Build history of the part. All positions in model axes, mm. Face numbers are marked on the shaded views. A direction names the side the tool comes from. Round coordinates to 2 decimals unless told otherwise and drop trailing zeros. Write each loop counter-clockwise with the first axis right and the second up, starting at its lowest first coordinate (ties: lowest second). Pieces come first, ordered by that corner, then holes. Notation, with made-up numbers: M 36.5,3 L 46.5,3 A31 cw 46.5,36 Z; hole C -24.75,-37.5 d2. An arc over 180 degrees is marked long. One line per item, written item: value. Start each with the question number.
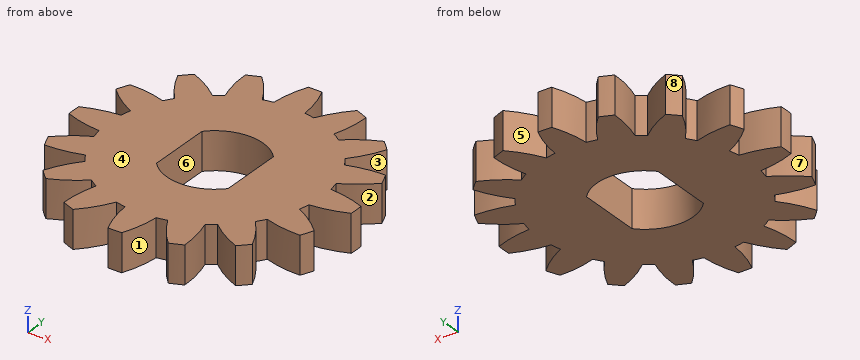
Autodesk Inventor part; units mm, degrees
ref_plane "YZ Plane" through (0, 0, 0) normal (1, 0, 0) x (0, 1, 0)
ref_plane "XZ Plane" through (0, 0, 0) normal (0, 1, 0) x (-1, 0, 0)
ref_plane "XY Plane" through (0, 0, 0) normal (0, 0, 1) x (1, 0, 0)
sketch "Sketch3" plane through (0, 0, 0) normal (0, 0, 1) x (1, 0, 0)
  arc A0 (12.7932, -14.1151) -> (14.1151, -12.7932) centre (0, 0) ccw
  arc A1 (14.1151, -12.7932) -> (11.4758, -8.5111) centre (-0.2655, -18.7022) ccw
  arc A2 (11.4758, -8.5111) -> (12.2548, -7.3452) centre (0, 0) ccw
  arc A3 (12.2548, -7.3452) -> (17.221, -8.1449) centre (17.177, 7.4023) ccw
  arc A4 (17.221, -8.1449) -> (17.9364, -6.4178) centre (0, 0) ccw
  arc A5 (17.9364, -6.4178) -> (13.8593, -3.4716) centre (6.9118, -17.3802) ccw
  arc A6 (13.8593, -3.4716) -> (14.1329, -2.0964) centre (0, 0) ccw
  arc A7 (14.1329, -2.0964) -> (19.0271, -0.9347) centre (13.0367, 13.4122) ccw
  arc A8 (19.0271, -0.9347) -> (19.0271, 0.9347) centre (0, 0) ccw
  arc A9 (19.0271, 0.9347) -> (14.1329, 2.0964) centre (13.0367, -13.4122) ccw
  arc A10 (14.1329, 2.0964) -> (13.8593, 3.4716) centre (0, 0) ccw
  arc A11 (13.8593, 3.4716) -> (17.9364, 6.4178) centre (6.9118, 17.3802) ccw
  arc A12 (17.9364, 6.4178) -> (17.221, 8.1449) centre (0, 0) ccw
  arc A13 (17.221, 8.1449) -> (12.2548, 7.3452) centre (17.177, -7.4023) ccw
  arc A14 (12.2548, 7.3452) -> (11.4758, 8.5111) centre (0, 0) ccw
  arc A15 (11.4758, 8.5111) -> (14.1151, 12.7932) centre (-0.2655, 18.7022) ccw
  arc A16 (14.1151, 12.7932) -> (12.7932, 14.1151) centre (0, 0) ccw
  arc A17 (12.7932, 14.1151) -> (8.5111, 11.4758) centre (18.7022, -0.2655) ccw
  arc A18 (8.5111, 11.4758) -> (7.3452, 12.2548) centre (0, 0) ccw
  arc A19 (7.3452, 12.2548) -> (8.1449, 17.221) centre (-7.4023, 17.177) ccw
  arc A20 (8.1449, 17.221) -> (6.4178, 17.9364) centre (0, 0) ccw
  arc A21 (6.4178, 17.9364) -> (3.4716, 13.8593) centre (17.3802, 6.9118) ccw
  arc A22 (3.4716, 13.8593) -> (2.0964, 14.1329) centre (0, 0) ccw
  arc A23 (2.0964, 14.1329) -> (0.9347, 19.0271) centre (-13.4122, 13.0367) ccw
  arc A24 (0.9347, 19.0271) -> (-0.9347, 19.0271) centre (0, 0) ccw
  arc A25 (-0.9347, 19.0271) -> (-2.0964, 14.1329) centre (13.4122, 13.0367) ccw
  arc A26 (-2.0964, 14.1329) -> (-3.4716, 13.8593) centre (0, 0) ccw
  arc A27 (-3.4716, 13.8593) -> (-6.4178, 17.9364) centre (-17.3802, 6.9118) ccw
  arc A28 (-6.4178, 17.9364) -> (-8.1449, 17.221) centre (0, 0) ccw
  arc A29 (-8.1449, 17.221) -> (-7.3452, 12.2548) centre (7.4023, 17.177) ccw
  arc A30 (-7.3452, 12.2548) -> (-8.5111, 11.4758) centre (0, 0) ccw
  arc A31 (-8.5111, 11.4758) -> (-12.7932, 14.1151) centre (-18.7022, -0.2655) ccw
  arc A32 (-12.7932, 14.1151) -> (-14.1151, 12.7932) centre (0, 0) ccw
  arc A33 (-14.1151, 12.7932) -> (-11.4758, 8.5111) centre (0.2655, 18.7022) ccw
  arc A34 (-11.4758, 8.5111) -> (-12.2548, 7.3452) centre (0, 0) ccw
  arc A35 (-12.2548, 7.3452) -> (-17.221, 8.1449) centre (-17.177, -7.4023) ccw
  arc A36 (-17.221, 8.1449) -> (-17.9364, 6.4178) centre (0, 0) ccw
  arc A37 (-17.9364, 6.4178) -> (-13.8593, 3.4716) centre (-6.9118, 17.3802) ccw
  arc A38 (-13.8593, 3.4716) -> (-14.1329, 2.0964) centre (0, 0) ccw
  arc A39 (-14.1329, 2.0964) -> (-19.0271, 0.9347) centre (-13.0367, -13.4122) ccw
  arc A40 (-19.0271, 0.9347) -> (-19.0271, -0.9347) centre (0, 0) ccw
  arc A41 (-19.0271, -0.9347) -> (-14.1329, -2.0964) centre (-13.0367, 13.4122) ccw
  arc A42 (-14.1329, -2.0964) -> (-13.8593, -3.4716) centre (0, 0) ccw
  arc A43 (-13.8593, -3.4716) -> (-17.9364, -6.4178) centre (-6.9118, -17.3802) ccw
  arc A44 (-17.9364, -6.4178) -> (-17.221, -8.1449) centre (0, 0) ccw
  arc A45 (-17.221, -8.1449) -> (-12.2548, -7.3452) centre (-17.177, 7.4023) ccw
  arc A46 (-12.2548, -7.3452) -> (-11.4758, -8.5111) centre (0, 0) ccw
  arc A47 (-11.4758, -8.5111) -> (-14.1151, -12.7932) centre (0.2655, -18.7022) ccw
  arc A48 (-14.1151, -12.7932) -> (-12.7932, -14.1151) centre (0, 0) ccw
  arc A49 (-12.7932, -14.1151) -> (-8.5111, -11.4758) centre (-18.7022, 0.2655) ccw
  arc A50 (-8.5111, -11.4758) -> (-7.3452, -12.2548) centre (0, 0) ccw
  arc A51 (-7.3452, -12.2548) -> (-8.1449, -17.221) centre (7.4023, -17.177) ccw
  arc A52 (-8.1449, -17.221) -> (-6.4178, -17.9364) centre (0, 0) ccw
  arc A53 (-6.4178, -17.9364) -> (-3.4716, -13.8593) centre (-17.3802, -6.9118) ccw
  arc A54 (-3.4716, -13.8593) -> (-2.0964, -14.1329) centre (0, 0) ccw
  arc A55 (-2.0964, -14.1329) -> (-0.9347, -19.0271) centre (13.4122, -13.0367) ccw
  arc A56 (-0.9347, -19.0271) -> (0.9347, -19.0271) centre (0, 0) ccw
  arc A57 (0.9347, -19.0271) -> (2.0964, -14.1329) centre (-13.4122, -13.0367) ccw
  arc A58 (2.0964, -14.1329) -> (3.4716, -13.8593) centre (0, 0) ccw
  arc A59 (3.4716, -13.8593) -> (6.4178, -17.9364) centre (17.3802, -6.9118) ccw
  arc A60 (6.4178, -17.9364) -> (8.1449, -17.221) centre (0, 0) ccw
  arc A61 (8.1449, -17.221) -> (7.3452, -12.2548) centre (-7.4023, -17.177) ccw
  arc A62 (7.3452, -12.2548) -> (8.5111, -11.4758) centre (0, 0) ccw
  arc A63 (8.5111, -11.4758) -> (12.7932, -14.1151) centre (18.7022, 0.2655) ccw
  circle A64 centre (0, 0) radius 16.9291 construction
  line L0 (-4.826, 4.3199) -> (-4.826, -4.3199)
  line L1 (4.826, 4.3199) -> (4.826, -4.3199)
  arc A65 (-4.826, -4.3199) -> (4.826, -4.3199) centre (0, 0) ccw
  arc A66 (4.826, 4.3199) -> (-4.826, 4.3199) centre (0, 0) ccw
  dimension "d14" = 19.05
  dimension "d15" = 33.8582
  dimension "d8" = 4.826
  dimension "d9" = 9.652
  dimension "d10" = 6.477
  dimension "d11" = 6.477
extrude "Extrusion2" add sketch "Sketch3" along normal blind 5.08
properties part number "Pinion"
Item 1: Cut at B-B, the plane y = -16. Write the cut outline in (x, z), plus the area to 3 significant figures.
Item 2: Cut at D-D, the plane x = 9. Write the cut outline in (y, z).
Item 3: Two-plate mould, pull along Y, no slides. Class the marked faces 1, 2, 3 and 4: pulls with the +Y half, pulls with the -Y half, needs draft (parallel to the pull), parting line crosses it, or undercut.
Item 4: Which spindle directions (+Z, -Z, +X, -X, +Y, -Y) get a long thin tool onto all of the face, cutting with end or side? Do the marked faces 5, 6, 7 and 8. Say none if no direction does.
Item 5: Drill centre lines: line 1 (Y direction, x = -16, z = 3.55); line 2 (X direction, y = -13, z = 0.3); line 3 (X direction, y = 12.5, z = 2.5). Where is each one in solid material? Low to high.
Item 6: Drop flat-ended pins along their axis: pin 1 (1.5 mm diameter, centred on y = -7, z = 2, fed in from -X); pin 2 (2.5 mm diameter, centred on y = 0.5, z = 1.5, fed in from +X); pin 3 (3 mm diameter, centred on x = 10, z = 3, fed in from +Y). Give the stop position or say it passes through.
Item 7: Cut at C-C, the plane y = 10. Write the cut outline in (x, z).
Item 8: Cut at A-A, the plane x = -4. Write the cut outline in (y, z).
Computed values:
1. outline: M -8.1,0 L -4.77,0 L -4.77,5.08 L -8.1,5.08 Z; M -1.85,0 L 1.85,0 L 1.85,5.08 L -1.85,5.08 Z; M 4.77,0 L 8.1,0 L 8.1,5.08 L 4.77,5.08 Z
1. area: 52.7 mm2
2. outline: M -11.88,0 L 11.88,0 L 11.88,5.08 L -11.88,5.08 Z
3. face 1: pulls with the -Y half
3. face 2: undercut
3. face 3: undercut
3. face 4: needs draft
4. face 5: +Z, -Z, +Y
4. face 6: +Z, -Z
4. face 7: +Z, -Z, -X
4. face 8: +Z, -Z, -X, +Y
5. line 1: y = -8.1 to -4.77, -1.85 to 1.85, 4.77 to 8.1
5. line 2: x = -13.92 to -10.59, -7.57 to 7.57, 10.59 to 13.92
5. line 3: x = -13.99 to -9.83, -7.42 to 7.42, 9.83 to 13.99
6. pin 1: stops at x = -17.94
6. pin 2: stops at x = 19.05
6. pin 3: stops at y = 13.51
7. outline: M -12.62,0 L 12.62,0 L 12.62,5.08 L -12.62,5.08 Z
8. outline: M -14.83,0 L -5.09,0 L -5.09,5.08 L -14.83,5.08 Z; M 5.09,0 L 14.83,0 L 14.83,5.08 L 5.09,5.08 Z
